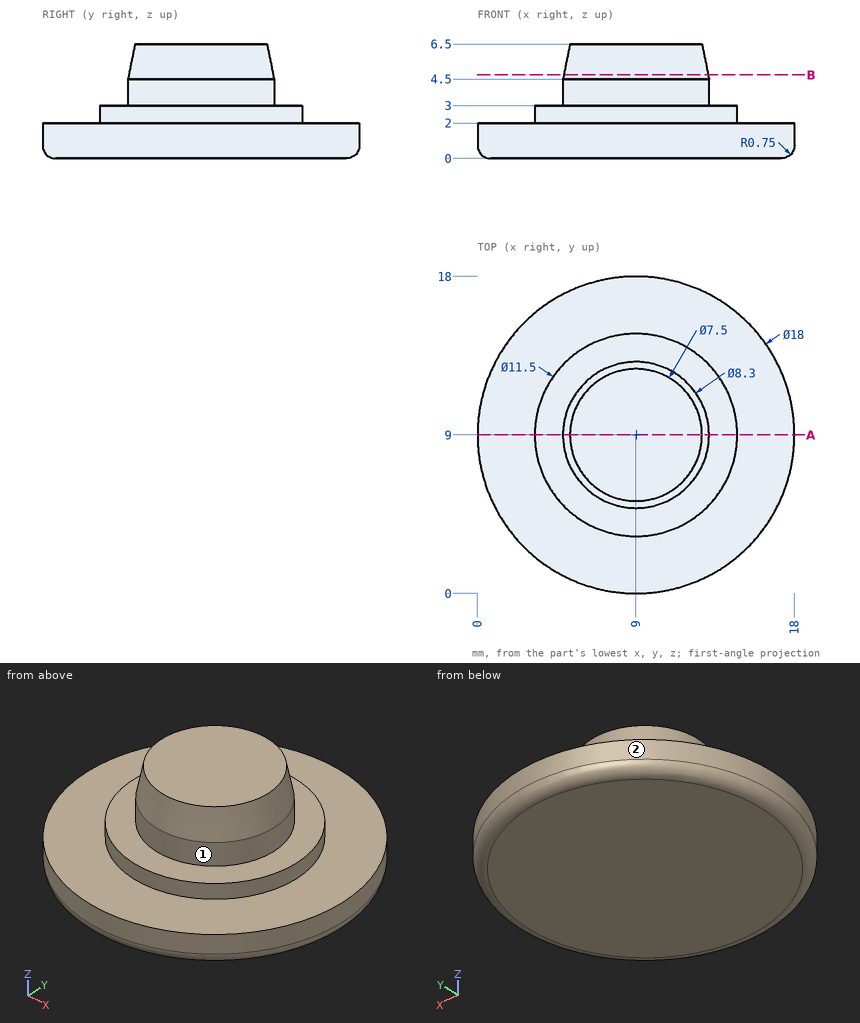
Geometry check sheet. Reference: drawing and pictorial views, mm from the part's lowest x, y, z. A direction names the side the tool comes from. Give positions to 0.01 mm unless a question says otherwise; leave off trailing zeros. Order: outer loops, then holes, each group sorted by start corner. A loop starts at its lowest first (then second) coordinate and runs counter-clockwise, first axis right, second up. Notation, with made-up numbers: M -22.5,88.5 L 16.5,88.5 A11 cw 16.5,96.5 Z; hole C -8.75,48.5 d5. An arc over 180 degrees is marked long. Answer as CSV lines item,"result". Start each with the question number.
Item 1: Thickness scan on line 1 (Z direction, x = 3.25, y = 13.25); line 2 (Z direction, x = 13.25, y = 12.25); line 3 (X direction, y = 1, z = 1.25). Record the ranges inside material, lowest first. Write a range as [from, to].
Item 2: Cross-section at B-B on z = 4.75. Enter the section's corners in (x, y).
Item 3: Cross-section at A-A on y = 9. Enter the section's corners in (x, z), plus the area to 3 significant figures.
Item 4: Gauge pin test, flat end, axial feed: P1, Ø5, axis at x = 6, y = 12.5, coming from the +Z side. Record the tip position at first contact, or that the pin passes through.
Item 5: Tool access check on the marked faces 1 and 2. Record the directions out of +Z, -Z, +X, -X, +Y, -Y that give a thin tool (end or side, any length) a straight path to the whole face; none if there is none.
Established:
1,line 1,"z = [0, 2]"
1,line 2,"z = [0, 3]"
1,line 3,"x = [4.88, 13.12]"
2,outline,"C 9,9 d8.2"
3,outline,"M 0,0.75 A0.75 ccw 0.75,0 L 17.25,0 A0.75 ccw 18,0.75 L 18,2 L 14.75,2 L 14.75,3 L 13.15,3 L 13.15,4.5 L 12.75,6.5 L 5.25,6.5 L 4.85,4.5 L 4.85,3 L 3.25,3 L 3.25,2 L 0,2 Z"
3,area,"75.5 mm^2"
4,P1,"stops at z = 6.5"
5,face 1,"+Z"
5,face 2,"+Z, -Z"
